from build123d import *

# Parameters (mm, degrees)
F0_R          = 16.51
F1_DEPTH      = 3.175
F2_R          = 16.51
F2_R_2        = 16.1925
F3_DEPTH      = 1.27
F4_R          = 1.016
F5_DEPTH      = 50.8
F5_DEPTH_BACK = 50.8


with BuildPart() as f1:
    # F0 (on Top) → F1 (new body)
    with BuildSketch(Plane.XY):
        Circle(F0_R)
    extrude(amount=F1_DEPTH)

    # F2 (on face) → F3 (join)
    with BuildSketch(Plane.XY.offset(3.175)):
        Circle(F2_R)
        Circle(F2_R_2, mode=Mode.SUBTRACT)
    extrude(amount=F3_DEPTH)

    # F4 (on Right) → F5 (join, two sides)
    with BuildSketch(Plane.YZ) as f5_sk:
        with Locations((0, 2.159)):
            Circle(F4_R)
    extrude(amount=F5_DEPTH)
    extrude(f5_sk.sketch, amount=-F5_DEPTH_BACK)


solid = f1.part
Part model, mm, in its own coordinate system. A direction names the side the tool comes from. Coordinates: 2 decimals unless noted, no trailing zeros. Loops run counter-clockwise (first coordinate to the right, second up) from the corner with the lowest first, then second, coordinate; pieces in that order, holes last. Notation, with made-up numbers: (27, 18) - (82, 18) arc R24 cw to (82, 32) - close; hole circle Ø5 at (13.25, 83.25). An arc over 180 degrees is marked (long way). Write each question's results on one line, items separated by ' | '. Start each with the question number.
Q1. Two-plate mould, pull along X, no slides. Class faces 4 (the flat face through (-50.8, 0, 2)), 5 (the cylindrical face through (-12.85, -9.85, 3.8)), 6 (the flat face through (0, 0, 0)): +X half, -X half, draft (parallel to the pull), parting line (faces both ways), or undercut.
Q2. Slice it at D-D on x = 33. Give the cut face in (y, z), and give its area (3 significant figures).
Q3. Probe line 1 along X through (y, z) = (0, 3.8); line 2 along Z through (x, y) = (-7.5, 8.5) (3 decimals). List the from-to ranges inside material, lowest first.
Q4. Slice it at C-C on x = -11. Give the cut face in (y, z) (3 decimals), and give its area (3 significant figures).
Q5. Which spindle directions (+Z, -Z, +X, -X, +Y, -Y) get a long thin tool onto all of the face, cutting with end or side? Do faces 1 (the flat face through (0, 0, 3.175)), 2 (the cylindrical face through (33.399, -0.22, 1.167)), 3 (the cylindrical face through (-33.399, -0.22, 1.167)). Say none if no direction does.
Q6. Drop flat-ended pins along their axis: pin 1 Ø1 at (x, z) = (-13.5, 3) entering from -Y; pin 2 Ø1 at (x, y) = (0.5, -9) entering from +Z (3 decimals); pin 3 Ø1 at (y, z) = (-5, 0.5) entering from +X. Give the stop position or say it passes through.
Answer:
1) face 4: -X half | face 5: undercut | face 6: draft
2) outline: circle Ø2.03 at (0, 2.16) | area: 3.24 mm2
3) line 1: x = -16.51 to -16.19, 16.19 to 16.51 | line 2: z = 0 to 3.175
4) outline: (-12.312, 0) - (12.312, 0) - (12.312, 4.445) - (11.883, 4.445) - (11.883, 3.175) - (-11.883, 3.175) - (-11.883, 4.445) - (-12.312, 4.445) - close | area: 79.3 mm2
5) face 1: +Z | face 2: +X | face 3: -X
6) pin 1: stops at y = -10.18 | pin 2: stops at z = 3.175 | pin 3: stops at x = 15.88
